Can you work these out from the drawing? Everything is in mm from the part's minimum corner. A direction names the side the tool comes from. Round coordinates to 2 decimals unless told otherwise and drop trailing zeros. Write each loop counter-clockwise with the first axis right and the second up, starting at its lowest first coordinate (ties: lowest second). Pieces come first, ordered by that corner, then holes. Notation, with made-up numbers: (-23.75, 24.5) -> (20.25, 24.5) arc R13 ccw to (20.25, 41.5) -> close; hole circle Ø9 at (31.25, 77.5). An arc over 180 degrees is marked (long way). One line per question, with ' | ' between items. Start each with the question number.
1. For pin 1 Ø4 at (y, z) = (11, 14.5) entering from -X; pin 2 Ø4.5 at (x, z) = (12.5, 5) entering from +Y, each with a flat end and sliding along its axis, tell me the tip position at first contact or that it passes through.
2. Imagine slicing it at A-A, the plane x = 12.5. List the corners of the cut face in (y, z) for me, and give its area (3 significant figures).
3. If I drill on line 1 along Z through (x, y) = (12.5, 1.6); line 2 along X through (y, z) = (3.05, 12.5); line 3 along Y through (x, z) = (1.5, 9.5), over which ranges is the centre line in solid material (lowest first)? Write a range as [from, to].
4. For the marked faces 1, 2 and 3, which set-ups out of +Z, -Z, +X, -X, +Y, -Y let a thin tool reach every point of the face, with its end or its side?
5. Imagine slicing it at C-C, the plane x = 5. List the corners of the cut face in (y, z) for me.
6. Imagine slicing it at B-B, the plane z = 12.5. List the corners of the cut face in (x, y) for me.
7. Thinking about a two-plate mould opening in X: for the marked faces 4, 5 and 6, which applies, released by +X, released by -X, zero draft, split by the parting line, or undercut?
8. Imagine slicing it at D-D, the plane z = 5. List the corners of the cut face in (x, y) for me.
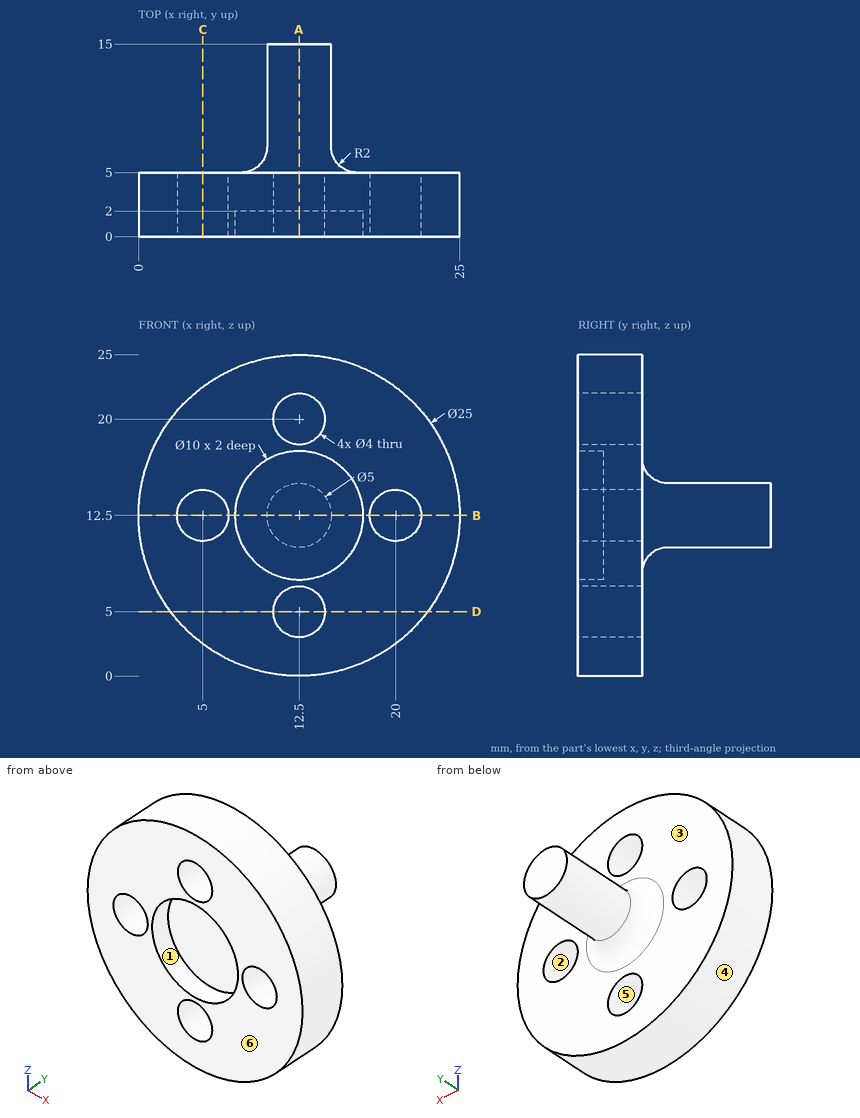
Geometry results:
1) pin 1: stops at x = 10 | pin 2: stops at y = 5
2) outline: (0, 0) -> (5, 0) -> (5, 3) -> (0, 3) -> close; (0, 7) -> (5, 7) -> (5, 8) arc R2 cw to (7, 10) -> (15, 10) -> (15, 15) -> (7, 15) arc R2 cw to (5, 17) -> (5, 18) -> (0, 18) -> (0, 17.5) -> (2, 17.5) -> (2, 7.5) -> (0, 7.5) -> close; (0, 22) -> (5, 22) -> (5, 25) -> (0, 25) -> close | area: 117 mm2
3) line 1: z = [0, 3], [7, 7.5], [17.5, 18], [22, 25] | line 2: x = [0, 3], [7, 18], [22, 25] | line 3: y = [0, 5]
4) face 1: -Y | face 2: +Y, -Y | face 3: +Y
5) outline: (0, 2.5) -> (5, 2.5) -> (5, 10.5) -> (0, 10.5) -> close; (0, 14.5) -> (5, 14.5) -> (5, 22.5) -> (0, 22.5) -> close
6) outline: (0, 0) -> (3, 0) -> (3, 5) -> (0, 5) -> close; (7, 0) -> (7.5, 0) -> (7.5, 2) -> (17.5, 2) -> (17.5, 0) -> (18, 0) -> (18, 5) -> (17, 5) arc R2 cw to (15, 7) -> (15, 15) -> (10, 15) -> (10, 7) arc R2 cw to (8, 5) -> (7, 5) -> close; (22, 0) -> (25, 0) -> (25, 5) -> (22, 5) -> close
7) face 4: split by the parting line | face 5: undercut | face 6: zero draft
8) outline: (2.5, 0) -> (10.5, 0) -> (10.5, 5) -> (2.5, 5) -> close; (14.5, 0) -> (22.5, 0) -> (22.5, 5) -> (14.5, 5) -> close
